Source: CAD feature listing. Evaluate the final solid. Frame: model axes, mm. A direction names the side the tool comes from. Coordinates: 2 decimals unless noted, no trailing zeros. Order: outer loops, then holes, each group sorted by start corner. A loop starts at its lowest first (then second) coordinate and runs counter-clockwise, first axis right, second up.
```python
from build123d import *

# Parameters (mm, degrees)
BOSS_EXTRUDE1_DEPTH = 1.5875
CUT_EXTRUDE1_REACH  = 97.488
SKETCH2_R           = 1.1303


with BuildPart() as part:
    # Sketch1 → Boss-Extrude1 (new body)
    with BuildSketch(Plane.XY):
        Polygon((91.44, 21.110587397), (91.44, 27.460587397), (0, 6.35), (0, 0), align=None)
    extrude(amount=BOSS_EXTRUDE1_DEPTH)

    # Sketch2 → Cut-Extrude1 (cut, up to next)
    with BuildSketch(Plane.XY.offset(1.5875), mode=Mode.PRIVATE) as cut_extrude1_sk1:
        with BuildLine():
            Line((3.4925, 0.806307158), (5.08, 1.172810411))
            Line((5.08, 1.172810411), (5.08, 4.347810411))
            ThreePointArc((5.08, 4.347810411), (4.102998373, 4.958308784), (3.4925, 3.981307158))
            Line((3.4925, 3.981307158), (3.4925, 0.806307158))
        make_face()
    cut_extrude1_tool1 = extrude(cut_extrude1_sk1.sketch, amount=-CUT_EXTRUDE1_REACH, mode=Mode.PRIVATE) & part.part
    # Sketch2 → Cut-Extrude1 (cut, up to next)
    with BuildSketch(Plane.XY.offset(1.5875), mode=Mode.PRIVATE) as cut_extrude1_sk2:
        with BuildLine():
            Line((91.44, 23.888712397), (91.44, 27.460587397))
            Line((91.44, 27.460587397), (89.8525, 27.094084143))
            Line((89.8525, 27.094084143), (89.8525, 24.682462397))
            ThreePointArc((89.8525, 24.682462397), (90.084983992, 24.121196389), (90.64625, 23.888712397))
            Line((90.64625, 23.888712397), (91.44, 23.888712397))
        make_face()
    cut_extrude1_tool2 = extrude(cut_extrude1_sk2.sketch, amount=-CUT_EXTRUDE1_REACH, mode=Mode.PRIVATE) & part.part
    # Sketch2 → Cut-Extrude1 (cut, up to next)
    with BuildSketch(Plane.XY.offset(1.5875), mode=Mode.PRIVATE) as cut_extrude1_sk3:
        with Locations((15.748, 6.810712274)):
            Circle(SKETCH2_R)
    cut_extrude1_tool3 = extrude(cut_extrude1_sk3.sketch, amount=-CUT_EXTRUDE1_REACH, mode=Mode.PRIVATE) & part.part
    # Sketch2 → Cut-Extrude1 (cut, up to next)
    with BuildSketch(Plane.XY.offset(1.5875), mode=Mode.PRIVATE) as cut_extrude1_sk4:
        with Locations((30.988, 10.329143507)):
            Circle(SKETCH2_R)
    cut_extrude1_tool4 = extrude(cut_extrude1_sk4.sketch, amount=-CUT_EXTRUDE1_REACH, mode=Mode.PRIVATE) & part.part
    add(cut_extrude1_tool1.solids().sort_by_distance((4.272922, 2.906844, 1.5875))[0], mode=Mode.SUBTRACT)
    add(cut_extrude1_tool2.solids().sort_by_distance((90.676821, 25.62383, 1.5875))[0], mode=Mode.SUBTRACT)
    add(cut_extrude1_tool3.solids().sort_by_distance((15.748, 6.810712, 1.5875))[0], mode=Mode.SUBTRACT)
    add(cut_extrude1_tool4.solids().sort_by_distance((30.988, 10.329144, 1.5875))[0], mode=Mode.SUBTRACT)


solid = part.part
```
1. Section query B-B, the plane x = 16. Output: boundary loops of the cut face in (y, z).
2. Section query A-A, the plane y = 3. Output: boundary loops of the cut face in (x, z), plus the area to 3 significant figures.
3. Section query D-D, the plane x = 68. Output: boundary loops of the cut face in (y, z), plus the area to 3 significant figures.
4. Access query for faces 1 (the flat face through (3.492, 2, 1)), 2 (the flat face through (89.852, 26, 1)), 3 (the flat face through (46, 14, 1.588)). Directions: +Z, -Z, +X, -X, +Y, -Y. A direction counts if a zero-diameter tool reaches every point of the face in a straight line with its end or side. Return the directions, or none.
5. Draft query along X for faces 4 (the flat face through (47.655, 11.002, 0.783)), 5 (the flat face through (45.56, 16.87, 0.78)), 6 (the flat face through (5.08, 3, 1)), 7 (the cylindrical face through (4.12, 4.96, 0.8)). Return one class per face: +X half, -X half, draft (parallel to the pull), parting line (faces both ways), or undercut.
6. Contact query for flat-ended pins moving along their axis: P1, Ø1.8, axis at x = 15.75, y = 6.81, coming from the -Z side; P2, Ø0.9, axis at x = 91, z = 0.5, coming from the +Y side. Output: stop coordinate, or through.
7. Material intervals for line 1 along Y through (x, z) = (86, 0.15); line 2 along Y through (x, z) = (42, 1.3), sorted ascending.
8. Section query C-C, the plane z = 0.8. Output: boundary loops of the cut face in (x, y).
Answer key:
1. outline: (3.69, 0) - (5.71, 0) - (5.71, 1.59) - (3.69, 1.59) - close; (7.91, 0) - (10.04, 0) - (10.04, 1.59) - (7.91, 1.59) - close
2. outline: (0, 0) - (3.49, 0) - (3.49, 1.59) - (0, 1.59) - close; (5.08, 0) - (12.99, 0) - (12.99, 1.59) - (5.08, 1.59) - close
2. area: 18.1 mm2
3. outline: (15.7, 0) - (22.05, 0) - (22.05, 1.59) - (15.7, 1.59) - close
3. area: 10.1 mm2
4. face 1: +Z, -Z, -Y
4. face 2: +Z, -Z, +X, +Y
4. face 3: +Z, +X, -X, +Y, -Y
5. face 4: +X half
5. face 5: -X half
5. face 6: undercut
5. face 7: undercut
6. P1: passes through
6. P2: stops at y = 23.89
7. line 1: y = 19.85 to 26.2
7. line 2: y = 9.7 to 16.05
8. outline: (0, 0) - (3.49, 0.81) - (3.49, 3.98) arc R0.81 cw to (5.08, 4.35) - (5.08, 1.17) - (91.44, 21.11) - (91.44, 23.89) - (90.65, 23.89) arc R0.79 cw to (89.85, 24.68) - (89.85, 27.09) - (0, 6.35) - close; hole circle Ø2.26 at (15.75, 6.81); hole circle Ø2.26 at (30.99, 10.33)
